Build history of the part. All positions in model axes, mm. Coordinates: 2 decimals unless noted, no trailing zeros. Loops run counter-clockwise (first coordinate to the right, second up) from the corner with the lowest first, then second, coordinate; pieces in that order, holes last. Notation, with made-up numbers: (5, 54) - (9, 54) arc R26 cw to (9, 68) - close; hole circle Ø9 at (59, 33). An arc over 180 degrees is marked (long way). One line per item, written item: value.
```python
from build123d import *

# Parameters (mm, degrees)
F1_DEPTH = 6


with BuildPart() as f1:
    # F0 (on Top) → F1 (new body)
    with BuildSketch(Plane.XY):
        with BuildLine():
            Line((99.539605, 94.727916), (-81.460395, 94.727916))
            ThreePointArc((-81.460395, 94.727916), (-83.581716, 93.849236), (-84.460395, 91.727916))
            Line((-84.460395, 91.727916), (-84.460395, -89.272084))
            ThreePointArc((-84.460395, -89.272084), (-83.581716, -91.393405), (-81.460395, -92.272084))
            Line((-81.460395, -92.272084), (99.539605, -92.272084))
            ThreePointArc((99.539605, -92.272084), (101.660925, -91.393405), (102.539605, -89.272084))
            Line((102.539605, -89.272084), (102.539605, 91.727916))
            ThreePointArc((102.539605, 91.727916), (101.660925, 93.849236), (99.539605, 94.727916))
        make_face()
        with BuildLine():
            ThreePointArc((9.615662, -54.603753), (7.269883, -61.770541), (6.141787, -69.226607))
            ThreePointArc((6.141787, -69.226607), (5.104101, -71.300549), (2.89785, -72.015028))
            ThreePointArc((2.89785, -72.015028), (-27.710395, -62.424951), (-51.319768, -40.712472))
            ThreePointArc((-51.319768, -40.712472), (-51.804137, -38.444562), (-50.526893, -36.508929))
            ThreePointArc((-50.526893, -36.508929), (-44.633798, -31.803936), (-39.600068, -26.189038))
            ThreePointArc((-39.600068, -26.189038), (-37.802948, -25.058948), (-35.707818, -25.401249))
            Line((-35.707818, -25.401249), (8.351782, -50.839072))
            ThreePointArc((8.351782, -50.839072), (9.695789, -52.482357), (9.615662, -54.603753))
        make_face(mode=Mode.SUBTRACT)
        with BuildLine():
            ThreePointArc((-55.480573, 30.775598), (-53.42718, 32.382849), (-50.891278, 31.775494))
            ThreePointArc((-50.891278, 31.775494), (-36.41773, -0.091822), (-52.990603, -30.919558))
            ThreePointArc((-52.990603, -30.919558), (-55.561454, -31.355915), (-57.502732, -29.614904))
            ThreePointArc((-57.502732, -29.614904), (-62.984472, 0.797757), (-55.480573, 30.775598))
        make_face(mode=Mode.SUBTRACT)
        with BuildLine():
            ThreePointArc((15.448073, -71.992174), (13.062505, -71.122238), (12.198598, -68.734479))
            ThreePointArc((12.198598, -68.734479), (31.757227, -38.120161), (68.049318, -36.489051))
            ThreePointArc((68.049318, -36.489051), (69.685225, -38.431095), (69.245828, -40.932026))
            ThreePointArc((69.245828, -40.932026), (45.789605, -62.424951), (15.448073, -71.992174))
        make_face(mode=Mode.SUBTRACT)
        with BuildLine():
            ThreePointArc((3.7593, -41.259398), (2.324711, -39.284367), (2.833078, -36.896825))
            ThreePointArc((2.833078, -36.896825), (21.402309, -20.184916), (45.159862, -12.459445))
            ThreePointArc((45.159862, -12.459445), (47.481717, -13.212957), (48.474849, -15.442863))
            Line((48.474849, -15.442863), (48.474849, -22.475358))
            ThreePointArc((48.474849, -22.475358), (47.704242, -24.482796), (45.788312, -25.458937))
            ThreePointArc((45.788312, -25.458937), (27.818105, -31.297402), (13.776743, -43.940825))
            ThreePointArc((13.776743, -43.940825), (11.973415, -45.111999), (9.84962, -44.775645))
            Line((9.84962, -44.775645), (3.7593, -41.259398))
        make_face(mode=Mode.SUBTRACT)
        with BuildLine():
            ThreePointArc((-1.726285, 35.423831), (19.144031, 17.022716), (45.735172, 8.832332))
            ThreePointArc((45.735172, 8.832332), (47.686293, 7.870842), (48.474849, 5.843648))
            Line((48.474849, 5.843648), (48.474849, -3.387817))
            ThreePointArc((48.474849, -3.387817), (47.686293, -5.415011), (45.735172, -6.376501))
            ThreePointArc((45.735172, -6.376501), (18.402309, -14.988763), (-2.722561, -34.353586))
            ThreePointArc((-2.722561, -34.353586), (-4.530796, -35.562562), (-6.680676, -35.231874))
            Line((-6.680676, -35.231874), (-14.675359, -30.616142))
            ThreePointArc((-14.675359, -30.616142), (-16.036683, -28.919635), (-15.893797, -26.749169))
            ThreePointArc((-15.893797, -26.749169), (-9.691308, 0.374626), (-15.191982, 27.649407))
            ThreePointArc((-15.191982, 27.649407), (-15.291169, 29.786156), (-13.941714, 31.445826))
            Line((-13.941714, 31.445826), (-5.639215, 36.239276))
            ThreePointArc((-5.639215, 36.239276), (-3.527171, 36.578104), (-1.726285, 35.423831))
        make_face(mode=Mode.SUBTRACT)
        with BuildLine():
            Line((54.474849, -24.209906), (54.474849, 26.665738))
            ThreePointArc((54.474849, 26.665738), (55.225973, 28.651325), (57.103219, 29.642631))
            ThreePointArc((57.103219, 29.642631), (64.482729, 31.19452), (71.50392, 33.945594))
            ThreePointArc((71.50392, 33.945594), (73.818849, 34.083902), (75.540732, 32.530472))
            ThreePointArc((75.540732, 32.530472), (82.539605, 1.227916), (75.540732, -30.074641))
            ThreePointArc((75.540732, -30.074641), (73.818849, -31.628071), (71.50392, -31.489762))
            ThreePointArc((71.50392, -31.489762), (64.482729, -28.738689), (57.103219, -27.186799))
            ThreePointArc((57.103219, -27.186799), (55.225973, -26.195493), (54.474849, -24.209906))
        make_face(mode=Mode.SUBTRACT)
        with BuildLine():
            ThreePointArc((-33.971698, 18.896247), (-34.051825, 21.017643), (-32.707818, 22.660928))
            Line((-32.707818, 22.660928), (-25.115336, 27.04445))
            ThreePointArc((-25.115336, 27.04445), (-22.687615, 27.299325), (-20.874126, 25.665295))
            ThreePointArc((-20.874126, 25.665295), (-15.685803, 1.227916), (-20.874126, -23.209464))
            ThreePointArc((-20.874126, -23.209464), (-22.687615, -24.843494), (-25.115336, -24.588619))
            Line((-25.115336, -24.588619), (-32.707818, -20.205097))
            ThreePointArc((-32.707818, -20.205097), (-34.051825, -18.561812), (-33.971698, -16.440416))
            ThreePointArc((-33.971698, -16.440416), (-30.39564, 1.227916), (-33.971698, 18.896247))
        make_face(mode=Mode.SUBTRACT)
        with BuildLine():
            ThreePointArc((-39.600068, 28.644869), (-43.965035, 33.61509), (-49.005428, 37.898835))
            ThreePointArc((-49.005428, 37.898835), (-50.187345, 39.792027), (-49.734823, 41.977509))
            ThreePointArc((-49.734823, 41.977509), (-27.029704, 63.944863), (2.799576, 74.351643))
            ThreePointArc((2.799576, 74.351643), (5.068332, 73.684327), (6.148737, 71.58069))
            ThreePointArc((6.148737, 71.58069), (7.281697, 64.176766), (9.615662, 57.059584))
            ThreePointArc((9.615662, 57.059584), (9.695789, 54.938188), (8.351782, 53.294903))
            Line((8.351782, 53.294903), (-35.707818, 27.857081))
            ThreePointArc((-35.707818, 27.857081), (-37.802948, 27.51478), (-39.600068, 28.644869))
        make_face(mode=Mode.SUBTRACT)
        with BuildLine():
            ThreePointArc((48.474849, 17.898695), (47.481717, 15.668789), (45.159862, 14.915277))
            ThreePointArc((45.159862, 14.915277), (22.460423, 22.04401), (4.301384, 37.417126))
            ThreePointArc((4.301384, 37.417126), (3.689978, 39.739023), (4.977435, 41.765714))
            Line((4.977435, 41.765714), (12.22419, 46.650974))
            ThreePointArc((12.22419, 46.650974), (14.341654, 47.130905), (16.228378, 46.056541))
            ThreePointArc((16.228378, 46.056541), (29.451174, 34.987266), (45.84648, 29.642631))
            ThreePointArc((45.84648, 29.642631), (47.723726, 28.651325), (48.474849, 26.665738))
            Line((48.474849, 26.665738), (48.474849, 17.898695))
        make_face(mode=Mode.SUBTRACT)
        with BuildLine():
            ThreePointArc((69.245828, 43.387857), (69.685225, 40.886926), (68.049318, 38.944882))
            ThreePointArc((68.049318, 38.944882), (31.757227, 40.575992), (12.198598, 71.19031))
            ThreePointArc((12.198598, 71.19031), (13.062505, 73.578069), (15.448073, 74.448005))
            ThreePointArc((15.448073, 74.448005), (45.789605, 64.880783), (69.245828, 43.387857))
        make_face(mode=Mode.SUBTRACT)
    extrude(amount=F1_DEPTH)


solid = f1.part
```
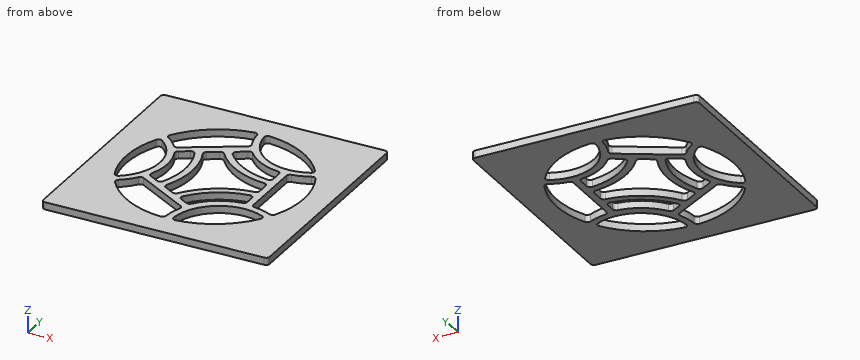
Item 1: Cut at B-B, the plane y = -58.5. Write the cut outline in (x, z), then the cut area to 3 significant figures.
Check result:
outline: (-84.46, 0) - (-33.8, 0) - (-33.8, 6) - (-84.46, 6) - close; (8.18, 0) - (14.52, 0) - (14.52, 6) - (8.18, 6) - close; (51.87, 0) - (102.54, 0) - (102.54, 6) - (51.87, 6) - close
area: 646 mm^2
Item 2: Probe probe 1 along Y at (x, z) = (73, 2.6); probe 2 along Y at (x, z) = (47.5, 1.9); probe 3 along Y at (x, z) = (43.5, 1.8). List the from-to ranges inside material, lowest first. Write a range as from..to.
Check result:
probe 1: y = -92.27..-31.79, 34.25..94.73
probe 2: y = -92.27..-61.41, -33.04..-24.69, -13.23..-5.6, 8.06..15.69, 28.88..35.49, 63.86..94.73
probe 3: y = -92.27..-63.69, -33.65..-25.76, -12.66..-6.61, 9.07..15.11, 30..36.11, 66.15..94.73
Item 3: Cut at C-C, the plane z = 4.3. Give the number of separate pieces and of enclosed holes in the cut face, then the cut area to 3 significant figures.
Check result:
separate pieces: 1
enclosed holes: 10
area: 22,100 mm^2
Item 4: Cut at A-A, the plane x = 32. Write the cut outline in (y, z), then the cut area to 3 significant figures.
Check result:
outline: (-92.27, 0) - (-68.59, 0) - (-68.59, 6) - (-92.27, 6) - close; (-37.98, 0) - (-29.16, 0) - (-29.16, 6) - (-37.98, 6) - close; (-15.37, 0) - (-9.06, 0) - (-9.06, 6) - (-15.37, 6) - close; (11.51, 0) - (17.82, 0) - (17.82, 6) - (11.51, 6) - close; (33.68, 0) - (40.44, 0) - (40.44, 6) - (33.68, 6) - close; (71.05, 0) - (94.73, 0) - (94.73, 6) - (71.05, 6) - close
area: 453 mm^2
